The model under review builds one solid part; all positions refer to its coordinate system, in mm. Coordinates: 2 decimals unless noted, no trailing zeros.
1) For line 1 (X direction, y = 22.5, z = -0.05); line 2 (X direction, y = 45, z = -0.1); line 3 (X direction, y = 39.5, z = -1.9), list the stretches that pass through material, from the lowest coordinate up.
2) Add section A-A, the plane z = -0.5. Give the number of separate pieces and of enclosed holes in the cut face, then the cut area to 3 significant figures.
3) For P1, Ø12, axis at x = -642, y = 47.5, coming from the +Z side, flat-tipped, find the tip position at first contact; note if it passes through.
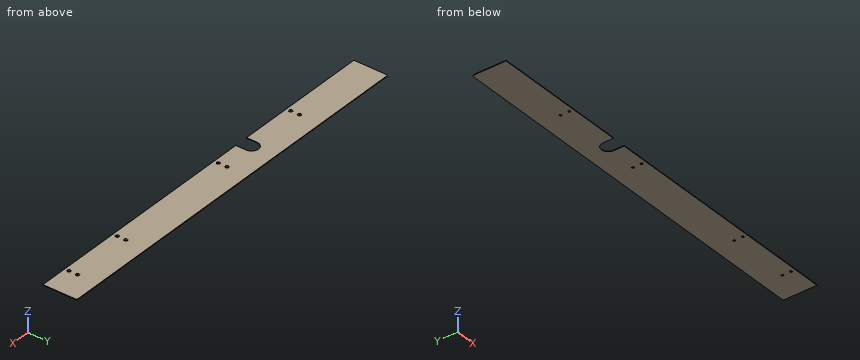
from build123d import *

# Parameters (mm, degrees)
F1_DEPTH       = 2
F2_D           = 5.5
F2_CSINK_D     = 11.2
F2_CSINK_ANGLE = 90


with BuildPart() as f1:
    # F0 (on Top) → F1 (new body)
    with BuildSketch(Plane.XY):
        with BuildLine():
            Line((-800, 0), (0, 0))
            Line((0, 0), (0, 105))
            ThreePointArc((0, 105), (-1.4644660941, 108.5355339059), (-5, 110))
            Line((-5, 110), (-1285, 110))
            ThreePointArc((-1285, 110), (-1288.5355339059, 108.5355339059), (-1290, 105))
            Line((-1290, 105), (-1290, 0))
            Line((-1290, 0), (-845, 0))
            Line((-845, 0), (-845, 33.5))
            ThreePointArc((-845, 33.5), (-822.5, 56), (-800, 33.5))
            Line((-800, 33.5), (-800, 0))
        make_face()
    extrude(amount=-F1_DEPTH)

    # F2 (through all)
    with Locations(Plane.XY):
        with Locations((-1010, 42), (-1010, 14), (-710, 42), (-710, 14), (-290, 42), (-290, 14), (-90, 42), (-90, 14)):
            CounterSinkHole(F2_D / 2, F2_CSINK_D / 2, counter_sink_angle=F2_CSINK_ANGLE)


solid = f1.part
Geometry results:
1. line 1: x = -1290 to -845, -800 to 0
1. line 2: x = -1290 to -1014.61, -1005.39 to -841.84, -803.16 to -714.61, -705.39 to -294.61, -285.39 to -94.61, -85.39 to 0
1. line 3: x = -1290 to -1012.73, -1007.27 to -844.19, -800.81 to -712.73, -707.27 to -292.73, -287.27 to -92.73, -87.27 to 0
2. separate pieces: 1
2. enclosed holes: 8
2. area: 139,000 mm2
3. P1: stops at z = 0
